```python
from build123d import *

# Parameters (mm, degrees)
F1_DEPTH = 25.4
F3_DEPTH = 12.7
F5_DEPTH = 12.7


with BuildPart() as f1:
    # F0 (on Front) → F1 (new body)
    with BuildSketch(Plane.XZ):
        Polygon((0, 31.75), (0, 0), (31.75, 0), (19.05, 31.75), align=None)
    extrude(amount=F1_DEPTH)

    # F2 (on face) → F3 (join)
    with BuildSketch(Plane.XZ.offset(25.4)):
        Polygon((19.05, 31.75), (31.75, 0), (57.15, 0), (44.45, 31.75), align=None)
    extrude(amount=-F3_DEPTH)

    # F4 (on face) → F5 (join)
    with BuildSketch(Plane.XZ.offset(25.4)):
        Polygon((0, 31.75), (0, 0), (28.575, 0), (19.05, 31.75), align=None)
    extrude(amount=F5_DEPTH)


solid = f1.part
```
Can you work these out from the model? Positions are in its coordinate system, mm. A direction names the side the tool comes from. Give positions to 0.01 mm unless a question says otherwise; leave off trailing zeros. Loops run counter-clockwise (first coordinate to the right, second up) from the corner with the lowest first, then second, coordinate; pieces in that order, holes last. Notation, with made-up numbers: M 40.5,31 L 73.5,31 A12 cw 73.5,41 Z; hole C 81,80.25 d3. An arc over 180 degrees is marked long. One line per question, with ' | ' between items. Start each with the question number.
Q1. If I drill on line 1 (Y direction, x = 41.5, z = 23); line 2 (X direction, y = -22.5, z = 1.5); line 3 (X direction, y = -18.5, z = 29.5), over which ranges is the centre line in solid material (lowest first)? Write a range as from..to.
Q2. For faces 4 (the flat face through (38, -25.4, 16)), 5 (the flat face through (25.49, -6.26, 15.65)), 6 (the flat face through (0, -19, 16)), which set-ups out of +Z, -Z, +X, -X, +Y, -Y let a thin tool reach every point of the face, with its end or its side?
Q3. For pin 1 Ø8 at (y, z) = (-29, 23.5) entering from +X; pin 2 Ø10 at (x, z) = (43.5, 14) entering from -Y; pin 3 Ø1.5 at (y, z) = (-17, 18) entering from +X, each with a flat end and sliding along its axis, tell me the tip position at first contact or that it passes through.
Q4. If we section it at C-C (x = 21): Please give me the cut outline in (y, z) (3 decimals).
Q5. If we section it at B-B (y = -27): Please give me the cut outline in (x, z) (3 decimals), plus the area to 3 significant figures.
Q6. If we section it at A-A (z = 25): Please give me the cut outline in (x, y) (3 decimals).
Q7. If we section it at D-D (y = -7): Please give me the cut outline in (x, z), plus the area to 3 significant figures.
Q8. If we mould it in two halves opening along Y, with no side actions, what happens to faces 1 (the flat face through (12, 0, 16)), 2 (the flat face through (23.88, -31.66, 15.65)), 3 (the flat face through (11, -38.1, 16))? For each: +Y half, -Y half, draft (parallel to the pull), parting line (faces both ways), or undercut.
Computed:
1) line 1: y = -25.4..-12.7 | line 2: x = 0..56.55 | line 3: x = 0..45.35
2) face 4: +Z, +X, -Y | face 5: +Z, +X, +Y | face 6: +Z, -Z, -X, +Y, -Y
3) pin 1: stops at x = 48.45 | pin 2: stops at y = -25.4 | pin 3: stops at x = 50.25
4) outline: M -38.1,0 L 0,0 L 0,26.875 L -12.7,26.875 L -12.7,31.75 L -25.4,31.75 L -25.4,25.25 L -38.1,25.25 Z
5) outline: M 0,0 L 28.575,0 L 19.05,31.75 L 0,31.75 Z | area: 756 mm²
6) outline: M 0,-38.1 L 21.075,-38.1 L 21.075,-25.4 L 47.15,-25.4 L 47.15,-12.7 L 21.75,-12.7 L 21.75,0 L 0,0 Z
7) outline: M 0,0 L 31.75,0 L 19.05,31.75 L 0,31.75 Z | area: 806 mm²
8) face 1: +Y half | face 2: draft | face 3: -Y half
